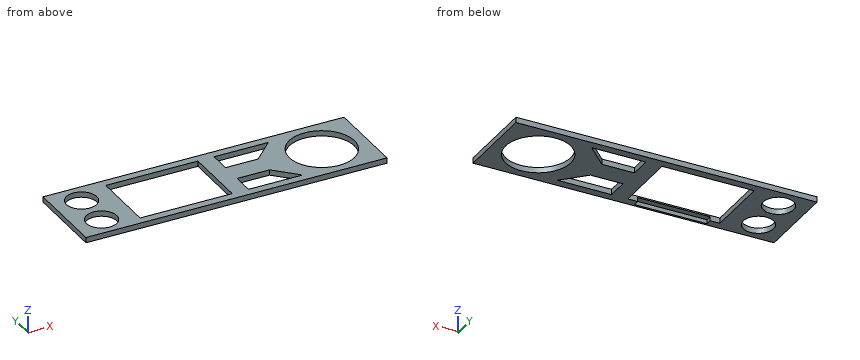
from build123d import *

# Parameters (mm, degrees)
SKETCH2_W           = 111.14
SKETCH2_H           = 30
SKETCH2_R           = 5.59
SKETCH2_R_2         = 12
SKETCH2_W_2         = 34
SKETCH2_H_2         = 24
BOSS_EXTRUDE1_DEPTH = 2
SKETCH3_W           = 26.7
SKETCH3_H           = 2.25
CUT_EXTRUDE1_DEPTH  = 1.5


with BuildPart() as part:
    # Sketch2 → Boss-Extrude1 (new body)
    with BuildSketch(Plane.XY):
        with Locations((-55.57, 15)):
            Rectangle(SKETCH2_W, SKETCH2_H)
        with Locations((-101.14, 22)):
            Circle(SKETCH2_R, mode=Mode.SUBTRACT)
        with Locations((-101.14, 8)):
            Circle(SKETCH2_R, mode=Mode.SUBTRACT)
        with Locations((-16.14, 15)):
            Circle(SKETCH2_R_2, mode=Mode.SUBTRACT)
        Polygon((-36.596, 27), (-29.55, 27), (-37.55, 19), (-49.55, 19), (-49.55, 27), align=None, mode=Mode.SUBTRACT)
        Polygon((-49.55, 3), (-37.006, 3), (-29.55, 3), (-37.55, 11), (-49.55, 11), align=None, mode=Mode.SUBTRACT)
        with Locations((-72.55, 15)):
            Rectangle(SKETCH2_W_2, SKETCH2_H_2, mode=Mode.SUBTRACT)
    extrude(amount=BOSS_EXTRUDE1_DEPTH)

    # Sketch3 → Cut-Extrude1 (cut)
    with BuildSketch(Plane(origin=(0, 0, 0), x_dir=(-1, 0, 0), z_dir=(0, 0, -1))):
        with Locations((72.55, 1.875)):
            Rectangle(SKETCH3_W, SKETCH3_H)
    extrude(amount=-CUT_EXTRUDE1_DEPTH, mode=Mode.SUBTRACT)


solid = part.part
Check sheet for the modelled part. Datum: model origin and axes. Units: mm. Round coordinates to 2 decimals unless told otherwise and drop trailing zeros. Loops run counter-clockwise (first coordinate to the right, second up) from the corner with the lowest first, then second, coordinate; pieces in that order, holes last.
1. Scan lines: probe 1 along Y at (x, z) = (-101.14, 0.95); probe 2 along Y at (x, z) = (-38, 0.4); probe 3 along Y at (x, z) = (-16.14, 0.6). Record each from-to range of solid material in increasing order.
2. Sectioned sample at D-D on z = 1.1. Record the boundary of the cut face in (x, y), and give its area (3 significant figures).
3. Sectioned sample at A-A on y = 15. Record the boundary of the cut face in (x, z), and give its area (3 significant figures).
4. Sectioned sample at B-B on x = -16.14. Record the boundary of the cut face in (y, z), and give its area (3 significant figures).
5. Sectioned sample at C-C on x = -40. Record the boundary of the cut face in (y, z), and give its area (3 significant figures).
Recorded:
1. probe 1: y = 0 to 2.41, 13.59 to 16.41, 27.59 to 30
1. probe 2: y = 0 to 3, 11 to 19, 27 to 30
1. probe 3: y = 0 to 3, 27 to 30
2. outline: (-111.14, 0) - (0, 0) - (0, 30) - (-111.14, 30) - close; hole circle Ø11.18 at (-101.14, 8); hole circle Ø11.18 at (-101.14, 22); hole (-89.55, 3) - (-85.9, 3) - (-85.9, 0.75) - (-59.2, 0.75) - (-59.2, 3) - (-55.55, 3) - (-55.55, 27) - (-89.55, 27) - close; hole (-49.55, 3) - (-29.55, 3) - (-37.55, 11) - (-49.55, 11) - close; hole (-49.55, 19) - (-37.55, 19) - (-29.55, 27) - (-49.55, 27) - close; hole circle Ø24 at (-16.14, 15)
2. area: 1,550 mm2
3. outline: (-111.14, 0) - (-89.55, 0) - (-89.55, 2) - (-111.14, 2) - close; (-55.55, 0) - (-28.14, 0) - (-28.14, 2) - (-55.55, 2) - close; (-4.14, 0) - (0, 0) - (0, 2) - (-4.14, 2) - close
3. area: 106 mm2
4. outline: (0, 0) - (3, 0) - (3, 2) - (0, 2) - close; (27, 0) - (30, 0) - (30, 2) - (27, 2) - close
4. area: 12.0 mm2
5. outline: (0, 0) - (3, 0) - (3, 2) - (0, 2) - close; (11, 0) - (19, 0) - (19, 2) - (11, 2) - close; (27, 0) - (30, 0) - (30, 2) - (27, 2) - close
5. area: 28.0 mm2
